Build history of the part. All positions in model axes, mm. A direction names the side the tool comes from. Round coordinates to 2 decimals unless told otherwise and drop trailing zeros. Write each loop counter-clockwise with the first axis right and the second up, starting at its lowest first coordinate (ties: lowest second). Pieces come first, ordered by that corner, then holes. Notation, with made-up numbers: (-18, -33.5) -> (25, -33.5) arc R25 ccw to (25, -8.5) -> close; hole circle Ø2 at (27.25, -12.5). An arc over 180 degrees is marked (long way). Return JSON: item names as keys, results as strings.
from build123d import *

# Parameters (mm, degrees)
F0_W     = 1524
F0_H     = 914.4
F1_DEPTH = 25.4
F2_W     = 1473.2
F2_H     = 863.6
F2_W_2   = 1371.6
F2_H_2   = 762
F3_DEPTH = 50.8
F4_W     = 50.8
F4_H     = 50.8
F5_DEPTH = 838.2
F6_W     = 50.8
F6_H     = 50.8
F7_DEPTH = 1371.6
F8_W     = 50.8
F8_H     = 50.8
F9_DEPTH = 762


with BuildPart() as f1:
    # F0 (on Top) → F1 (new body)
    with BuildSketch(Plane.XY):
        Rectangle(F0_W, F0_H)
    extrude(amount=-F1_DEPTH)

    # F2 (on face) → F3 (join)
    with BuildSketch(Plane(origin=(0, 0, -25.4), x_dir=(1, 0, 0), z_dir=(0, 0, -1))):
        Rectangle(F2_W, F2_H)
        Rectangle(F2_W_2, F2_H_2, mode=Mode.SUBTRACT)
    extrude(amount=F3_DEPTH)

    # F4 (on face) → F5 (join)
    with BuildSketch(Plane(origin=(0, 0, -76.2), x_dir=(1, 0, 0), z_dir=(0, 0, -1))):
        with Locations((711.2, 406.4)):
            Rectangle(F4_W, F4_H)
        with Locations((711.2, -406.4)):
            Rectangle(F4_W, F4_H)
        with Locations((-711.2, -406.4)):
            Rectangle(F4_W, F4_H)
        with Locations((-711.2, 406.4)):
            Rectangle(F4_W, F4_H)
    extrude(amount=F5_DEPTH)

    # F6 (on face) → F7 (join, through all)
    with BuildSketch(Plane.YZ.offset(-685.8)):
        with Locations((-406.4, -685.8)):
            Rectangle(F6_W, F6_H)
    extrude(amount=F7_DEPTH)

    # F8 (on face) → F9 (join, through all)
    with BuildSketch(Plane(origin=(0, -381, 0), x_dir=(-1, 0, 0), z_dir=(0, 1, 0))):
        with Locations((-711.2, -685.8)):
            Rectangle(F8_W, F8_H)
        with Locations((711.2, -685.8)):
            Rectangle(F8_W, F8_H)
    extrude(amount=F9_DEPTH)


solid = f1.part
Q1. Two-plate mould, pull along Z, no slides. Class faces 1 (the flat face through (-712, -381, -364)), 2 (the flat face through (685.8, 5, -50)), 3 (the flat face through (-712, 406, -914.4)): +Z half, -Z half, draft (parallel to the pull), parting line (faces both ways), or undercut.
Verdict:
{"face 1": "undercut", "face 2": "draft", "face 3": "-Z half"}
Q2. Saw through at C-C on x = -47.5. List the corners of the cut face in (y, z).
Verdict:
{"outline": "(-457.2, -25.4) -> (-431.8, -25.4) -> (-431.8, -76.2) -> (-381, -76.2) -> (-381, -25.4) -> (381, -25.4) -> (381, -76.2) -> (431.8, -76.2) -> (431.8, -25.4) -> (457.2, -25.4) -> (457.2, 0) -> (-457.2, 0) -> close; (-431.8, -711.2) -> (-381, -711.2) -> (-381, -660.4) -> (-431.8, -660.4) -> close"}
Q3. Saw through at A-A on z = -259. List the corners of the cut face in (x, y).
Verdict:
{"outline": "(-736.6, -431.8) -> (-685.8, -431.8) -> (-685.8, -381) -> (-736.6, -381) -> close; (-736.6, 381) -> (-685.8, 381) -> (-685.8, 431.8) -> (-736.6, 431.8) -> close; (685.8, -431.8) -> (736.6, -431.8) -> (736.6, -381) -> (685.8, -381) -> close; (685.8, 381) -> (736.6, 381) -> (736.6, 431.8) -> (685.8, 431.8) -> close"}
Q4. Saw through at B-B on y = -153.5. List the corners of the cut face in (x, z).
Verdict:
{"outline": "(-762, -25.4) -> (-736.6, -25.4) -> (-736.6, -76.2) -> (-685.8, -76.2) -> (-685.8, -25.4) -> (685.8, -25.4) -> (685.8, -76.2) -> (736.6, -76.2) -> (736.6, -25.4) -> (762, -25.4) -> (762, 0) -> (-762, 0) -> close; (-736.6, -711.2) -> (-685.8, -711.2) -> (-685.8, -660.4) -> (-736.6, -660.4) -> close; (685.8, -711.2) -> (736.6, -711.2) -> (736.6, -660.4) -> (685.8, -660.4) -> close"}
Q5. Pin check, flat tips, straight feed: pin 1 Ø5 at (x, y) = (161, -239.5) entering from +Z; pin 2 Ø5 at (x, z) = (359, -698.5) entering from +Y; pin 3 Ø5 at (y, z) = (-128, -689.5) entering from -X. Stop position of each tip, or through.
Verdict:
{"pin 1": "stops at z = 0", "pin 2": "stops at y = -381", "pin 3": "stops at x = -736.6"}
Q6. Wall check: L1, parallel to X at y = 200, z = -67.5; L2, parallel to Y at x = 415.5, z = -68; L3, parallel to Z at x = 359, y = -398. Give the ranges that are in metal, low to high.
Verdict:
{"L1": "x = -736.6 to -685.8, 685.8 to 736.6", "L2": "y = -431.8 to -381, 381 to 431.8", "L3": "z = -711.2 to -660.4, -76.2 to 0"}
Q7. 3-axis set-ups, long thin cutter, end or side, ignore diameter. For faces 4 (the flat face through (711, 381, -811)), 5 (the flat face through (-711, -5, -660.4)), 6 (the flat face through (-685.8, -406, -811)): which of +Z, -Z, +X, -X, +Y, -Y reach the whole face in a straight line?
Verdict:
{"face 4": "-Z, +X, -X", "face 5": "+X, -X", "face 6": "-Z, +Y, -Y"}
Q8. Saw through at D-D on y = 398.5. List the corners of the cut face in (x, z).
Verdict:
{"outline": "(-762, -25.4) -> (-736.6, -25.4) -> (-736.6, -914.4) -> (-685.8, -914.4) -> (-685.8, -76.2) -> (685.8, -76.2) -> (685.8, -914.4) -> (736.6, -914.4) -> (736.6, -25.4) -> (762, -25.4) -> (762, 0) -> (-762, 0) -> close"}
